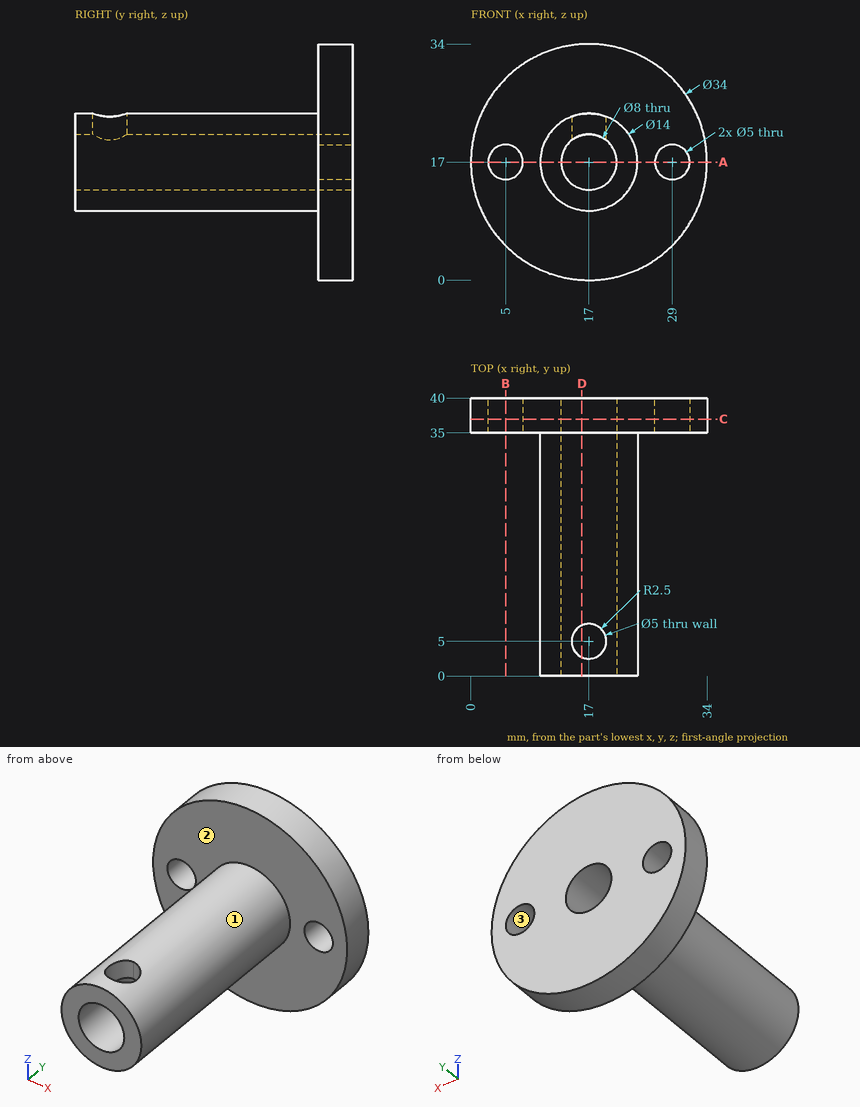
Geometry check sheet. Reference: drawing and pictorial views, mm from the part's lowest x, y, z. Coordinates: 2 decimals unless noted, no trailing zeros. Order: outer loops, then holes, each group sorted by start corner. A loop starts at its lowest first (then second) coordinate and runs counter-clockwise, first axis right, second up.
1. Sectioned sample at B-B, the plane x = 5. Record the cut outline in (y, z).
Results found:
outline: (35, 4.96) - (40, 4.96) - (40, 14.5) - (35, 14.5) - close; (35, 19.5) - (40, 19.5) - (40, 29.04) - (35, 29.04) - close
2. Go/stop test with flat-tipped pins: pin 1 Ø12 at (y, z) = (16, 6) entering from -X; pin 2 Ø12 at (x, y) = (5.5, 8) entering from -Z; pin 3 Ø12 at (y, z) = (13, 21) entering from +X; pin 4 Ø17 at (x, z) = (17.5, 13.5) entering from -Y. Record where each tip stops, or that it passes through.
Results found:
pin 1: stops at x = 12.1
pin 2: stops at z = 12.67
pin 3: stops at x = 24
pin 4: stops at y = 0
3. Sectioned sample at D-D, the plane x = 16. Record the cut outline in (y, z), and give its area (3 significant figures).
Results found:
outline: (0, 10.07) - (35, 10.07) - (35, 0.03) - (40, 0.03) - (40, 13.13) - (0, 13.13) - close; (0, 20.87) - (2.71, 20.87) - (2.71, 23.93) - (0, 23.93) - close; (7.29, 20.87) - (40, 20.87) - (40, 33.97) - (35, 33.97) - (35, 23.93) - (7.29, 23.93) - close
area: 331 mm2
4. Sectioned sample at C-C, the plane y = 37. Record the cut outline in (x, z).
Results found:
outline: circle Ø34 at (17, 17); hole circle Ø5 at (5, 17); hole circle Ø8 at (17, 17); hole circle Ø5 at (29, 17)
5. Release check for a two-part mould opening along Z. For the marked faces 1, 2 and 3 record: +Z half, -Z half, draft (parallel to the pull), parting line (faces both ways), or undercut.
Results found:
face 1: parting line
face 2: draft
face 3: undercut
6. Sectioned sample at A-A, the plane z = 17. Record the cut outline in (x, y).
Results found:
outline: (0, 35) - (2.5, 35) - (2.5, 40) - (0, 40) - close; (7.5, 35) - (10, 35) - (10, 0) - (13, 0) - (13, 40) - (7.5, 40) - close; (21, 0) - (24, 0) - (24, 35) - (26.5, 35) - (26.5, 40) - (21, 40) - close; (31.5, 35) - (34, 35) - (34, 40) - (31.5, 40) - close
7. Scan lines: line 1 (Z direction, x = 17, y = 18.5); line 2 (Y direction, x = 17, z = 23.25); line 3 (X direction, y = 6, z = 20). Record each from-to range of solid material in increasing order.
Results found:
line 1: z = 10 to 13, 21 to 24
line 2: y = 0 to 2.5, 7.5 to 40
line 3: x = 10.68 to 14.35, 19.65 to 23.32
